```python
from build123d import *

# Parameters (mm, degrees)
F0_R     = 1.75
F1_DEPTH = 10
F2_R     = 40
F3_R     = 35


with BuildPart() as f1:
    # F0 (on Top) → F1 (new body)
    with BuildSketch(Plane.XY):
        with BuildLine():
            Line((53, 0), (0, 0))
            Line((0, 0), (-53, 0))
            Line((-53, 0), (-74.842291, -5.861044))
            ThreePointArc((-74.842291, -5.861044), (-77.063211, -10.085928), (-72.677128, -11.968587))
            Line((-72.677128, -11.968587), (-53, -3.2))
            Line((-53, -3.2), (0, -3.2))
            Line((0, -3.2), (53, -3.2))
            Line((53, -3.2), (72.677128, -11.968587))
            ThreePointArc((72.677128, -11.968587), (77.063211, -10.085928), (74.842291, -5.861044))
            Line((74.842291, -5.861044), (53, 0))
        make_face()
        with Locations((-74, -9)):
            Circle(F0_R, mode=Mode.SUBTRACT)
        with Locations((74, -9)):
            Circle(F0_R, mode=Mode.SUBTRACT)
    extrude(amount=F1_DEPTH)

    # F2
    f2_edges = [f1.edges().sort_by_distance(p)[0] for p in [
        (53, 0, 5),
        (-53, 0, 5),
    ]]
    fillet(f2_edges, radius=F2_R)

    # F3
    f3_edges = [f1.edges().sort_by_distance(p)[0] for p in [
        (-53, -3.2, 5),
        (53, -3.2, 5),
    ]]
    fillet(f3_edges, radius=F3_R)


solid = f1.part
```
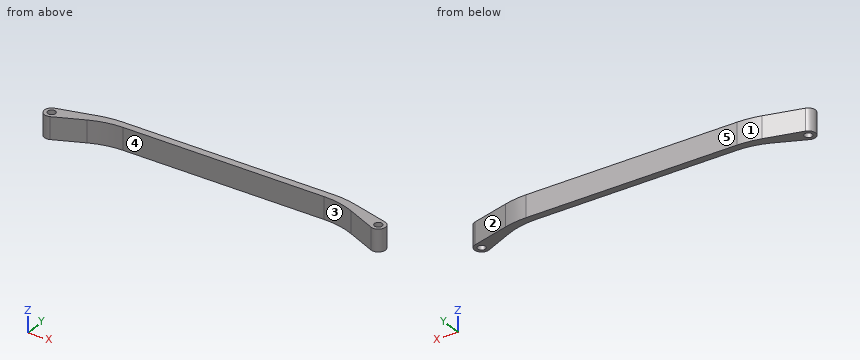
The model under review builds one solid part; all positions refer to its coordinate system, in mm. Face numbers are marked on the shaded views. A direction names the side the tool comes from. Round coordinates to 2 decimals unless told otherwise and drop trailing zeros. Loops run counter-clockwise (first coordinate to the right, second up) from the corner with the lowest first, then second, coordinate; pieces in that order, holes last. Notation, with made-up numbers: (-17.75, 46) -> (32.25, 46) arc R26 cw to (32.25, 69) -> close; hole circle Ø10 at (-27.75, 48). An arc over 180 degrees is marked (long way). Answer as a JSON object with one key per item and string values. Group by question number.
1) We need section A-A on z = 6. Write out the cut boundary in (x, y), then the cut area to 3 significant figures.
2) For the marked faces 4 and 5, list the 3-axis set-ups (+Z, -Z, +X, -X, +Y, -Y) from which the entire face can be reached by the end or side of a thin tool; tool diameter is ignored.
3) For pin 1 Ø5 at (x, z) = (-37, 5.5) entering from -Y; pin 2 Ø3 at (y, z) = (-10, 3.5) entering from +X, all flat-tipped, find the tip position at first contact; note any pin that passes through.
4) We need section B-B on y = -9. Write out the cut boundary in (x, z), then the cut area to 3 significant figures.
5) We need section D-D on x = 50.5. Write out the cut boundary in (y, z), then the cut area to 3 significant figures.
6) We need section C-C on x = 2. Write out the cut boundary in (y, z).
7) For line 1 (X direction, y = -9.25, z = 3.75); line 2 (Y direction, x = -12, z = 7); line 3 (Y direction, x = -74, z = 2), list the stretches that pass through material, from the lowest coordinate up. Write a range as [from, to].
8) Mouldability with a two-part tool opening along X and no side actions: class the marked faces 1, 2 and 3 as released by +X, released by -X, zero draft, split by the parting line, or undercut.
Result set:
{
 "1": {"outline": "(-74.84, -5.86) arc R3.25 ccw (long way) to (-72.68, -11.97) -> (-59.8, -6.23) arc R35 cw to (-45.55, -3.2) -> (45.55, -3.2) arc R35 cw to (59.8, -6.23) -> (72.68, -11.97) arc R3.25 ccw (long way) to (74.84, -5.86) -> (58.09, -1.37) arc R40 ccw to (47.73, 0) -> (-47.73, 0) arc R40 ccw to (-58.09, -1.37) -> close; hole circle Ø3.5 at (-74, -9); hole circle Ø3.5 at (74, -9)", "area": "571 mm²"},
 "2": {"face 4": "+Z, -Z, -Y", "face 5": "+Z, -Z, +X, -X, +Y"},
 "3": {"pin 1": "y = -3.2", "pin 2": "x = 77.25"},
 "4": {"outline": "(-77.25, 0) -> (-75.75, 0) -> (-75.75, 10) -> (-77.25, 10) -> close; (-72.25, 0) -> (-66.02, 0) -> (-66.02, 10) -> (-72.25, 10) -> close; (66.02, 0) -> (72.25, 0) -> (72.25, 10) -> (66.02, 10) -> close; (75.75, 0) -> (77.25, 0) -> (77.25, 10) -> (75.75, 10) -> close", "area": "155 mm²"},
 "5": {"outline": "(-3.55, 0) -> (-0.1, 0) -> (-0.1, 10) -> (-3.55, 10) -> close", "area": "34.5 mm²"},
 "6": {"outline": "(-3.2, 0) -> (0, 0) -> (0, 10) -> (-3.2, 10) -> close"},
 "7": {"line 1": "[-77.24, -75.73], [-72.27, -66.58], [66.58, 72.27], [75.73, 77.24]", "line 2": "[-3.2, 0]", "line 3": "[-12.25, -10.75], [-7.25, -5.64]"},
 "8": {"face 1": "released by -X", "face 2": "released by +X", "face 3": "undercut"}
}
